```python
from build123d import *

# Parameters (mm, degrees)
SKETCH_1_R          = 22.1
EXTRUDE_1_DEPTH     = 66.6
SKETCH_2_R          = 2.5
EXTRUDE_2_DEPTH     = 16.5
EXTRUDE_START       = 5
SKETCH_3_R          = 2.5
EXTRUDE_3_DEPTH     = 5
SKETCH_4_R          = 1.25
CUT_EXTRUDE_1_DEPTH = 5


with BuildPart() as part:
    # 草圖1 → 填料-伸長1 (new body)
    with BuildSketch(Plane(origin=(0, 0, 0), x_dir=(1, 0, 0), z_dir=(0, 1, 0))):
        with Locations(Location((0, 0, 0), (0, 0, 270))):
            Circle(SKETCH_1_R)
    extrude(amount=EXTRUDE_1_DEPTH)

    # 草圖2 → 填料-伸長2 (add)
    with BuildSketch(Plane(origin=(0, 66.6, 0), x_dir=(1, 0, 0), z_dir=(0, 1, 0))):
        with Locations(Location((0, 0, 0), (0, 0, 270))):
            Circle(SKETCH_2_R)
    extrude(amount=EXTRUDE_2_DEPTH)

    # 草圖3 → 填料-伸長3 (add)
    with BuildSketch(Plane.XZ.offset(EXTRUDE_START)):
        with Locations(Location((0, 0, 0), (0, 0, 90))):
            Circle(SKETCH_3_R)
    extrude(amount=-EXTRUDE_3_DEPTH)

    # 草圖4 → 除料-伸長1 (cut)
    with BuildSketch(Plane(origin=(0, 66.6, 0), x_dir=(1, 0, 0), z_dir=(0, 1, 0))):
        with Locations(Location((-16.165, 0, 0), (0, 0, 270))):
            Circle(SKETCH_4_R)
        with Locations(Location((16.165, 0, 0), (0, 0, 270))):
            Circle(SKETCH_4_R)
    extrude(amount=-CUT_EXTRUDE_1_DEPTH, mode=Mode.SUBTRACT)


solid = part.part
```
Source: CAD feature listing. Evaluate the final solid. Frame: model axes, mm. A direction names the side the tool comes from. Give positions to 0.01 mm unless a question says otherwise; leave off trailing zeros. Loops run counter-clockwise (first coordinate to the right, second up) from the corner with the lowest first, then second, coordinate; pieces in that order, holes last. Notation, with made-up numbers: (69, 5) - (104, 5) arc R28 cw to (104, 27) - close; hole circle Ø8 at (73, 10.5). An arc over 180 degrees is marked (long way). Use CSV: the item, a comma, the result in double quotes.
1) Cut plane C-C (y = 29). Output: boundary loops of the cut face in (x, z).
Worked out:
outline,"circle Ø44.2 at (0, 0)"
2) Line query: line 1 (X direction, y = 64, z = 0) (3 decimals); line 2 (Y direction, x = -8, z = -15); line 3 (X direction, y = 38, z = 7). Output: solid intervals per line, ascending.
Worked out:
line 1,"x = -22.1 to -17.415, -14.915 to 14.915, 17.415 to 22.1"
line 2,"y = 0 to 66.6"
line 3,"x = -20.96 to 20.96"
3) Pin query (flat end, axial travel): P1, Ø13.5, axis at x = -2.5, z = -3.5, coming from the -Y side; P2, Ø1.5, axis at x = -16.165, z = 0, coming from the -Y side; P3, Ø2, axis at x = 16, z = 0.5, coming from the +Y side; P4, Ø5, axis at y = 56.5, z = -16, coming from the +X side. Return the tip coordinate at first contact, or that it passes through.
Worked out:
P1,"stops at y = -5"
P2,"stops at y = 0"
P3,"stops at y = 66.6"
P4,"stops at x = 17.5"
4) Set-up query: faces 1 (the cylindrical face through (2.44, -2.54, -0.54)), 2 (the flat face through (-16, 61.6, 0)), 3 (the flat face through (0, -5, 0)). Return all of +Z, -Z, +X, -X, +Y, -Y with unobstructed straight access to the full face (end or side cutting, diameter ignored); none if empty.
Worked out:
face 1,"-Y"
face 2,"+Y"
face 3,"+Z, -Z, +X, -X, -Y"
5) Cut plane B-B (x = 0). Output: boundary loops of the cut face in (y, z), and give its area (3 significant figures).
Worked out:
outline,"(-5, -2.5) - (0, -2.5) - (0, -22.1) - (66.6, -22.1) - (66.6, -2.5) - (83.1, -2.5) - (83.1, 2.5) - (66.6, 2.5) - (66.6, 22.1) - (0, 22.1) - (0, 2.5) - (-5, 2.5) - close"
area,"3,050 mm^2"
6) Mould query, pull axis Z, two halves, no side actions, for faces 4 (the cylindrical face through (-21.574, 32.834, -4.791)), 5 (the flat face through (-5, 66.6, 0)), 6 (the cylindrical face through (-14.926, 64.135, -0.163)). Classes: +Z half, -Z half, draft (parallel to the pull), parting line (faces both ways), or undercut.
Worked out:
face 4,"parting line"
face 5,"draft"
face 6,"undercut"
7) Cut plane D-D (z = -5). Output: boundary loops of the cut face in (x, y), and give its area (3 significant figures).
Worked out:
outline,"(-21.53, 0) - (21.53, 0) - (21.53, 66.6) - (-21.53, 66.6) - close"
area,"2,870 mm^2"
8) Cut plane A-A (z = 0). Output: boundary loops of the cut face in (x, y) (3 decimals), and give its area (3 significant figures).
Worked out:
outline,"(-22.1, 0) - (-2.5, 0) - (-2.5, -5) - (2.5, -5) - (2.5, 0) - (22.1, 0) - (22.1, 66.6) - (17.415, 66.6) - (17.415, 61.6) - (14.915, 61.6) - (14.915, 66.6) - (2.5, 66.6) - (2.5, 83.1) - (-2.5, 83.1) - (-2.5, 66.6) - (-14.915, 66.6) - (-14.915, 61.6) - (-17.415, 61.6) - (-17.415, 66.6) - (-22.1, 66.6) - close"
area,"3,030 mm^2"
